Here's how the part is built. I have some questions about the finished solid (model axes, mm). Round coordinates to 2 decimals unless told otherwise and drop trailing zeros. Write each loop counter-clockwise with the first axis right and the second up, starting at its lowest first coordinate (ties: lowest second). Pieces come first, ordered by that corner, then holes. Notation, with made-up numbers: (-38.5, 57.25) - (1.5, 57.25) arc R32 ccw to (1.5, 83.25) - close; hole circle Ø11 at (-35, 54). An arc over 180 degrees is marked (long way). Return JSON: item names as keys, results as strings. Group by question number.
```python
from build123d import *

# Parameters (mm, degrees)
CROQUIS1_W              = 30
CROQUIS1_H              = 15
CROQUIS1_R              = 2.3
SALIENTE_EXTRUIR1_DEPTH = 16
CROQUIS2_W              = 120
CROQUIS2_H              = 50
CROQUIS2_R              = 3.5
SALIENTE_EXTRUIR2_DEPTH = 5
CROQUIS3_W              = 40
CROQUIS3_H              = 25
CROQUIS3_W_2            = 30
CROQUIS3_H_2            = 15
SALIENTE_EXTRUIR3_DEPTH = 4
CORTAR_EXTRUIR1_DEPTH   = 5
REDONDEO1_R             = 2


with BuildPart() as part:
    # Croquis1 → Saliente-Extruir1 (new body)
    with BuildSketch(Plane.XY):
        Rectangle(CROQUIS1_W, CROQUIS1_H)
        with Locations((6, 0)):
            Circle(CROQUIS1_R, mode=Mode.SUBTRACT)
        with Locations(Location((-6, 0, 0), (0, 0, 180))):
            Circle(CROQUIS1_R, mode=Mode.SUBTRACT)
    extrude(amount=SALIENTE_EXTRUIR1_DEPTH)

    # Croquis2 → Saliente-Extruir2 (add)
    with BuildSketch(Plane(origin=(0, 0, 0), x_dir=(-1, 0, 0), z_dir=(0, 0, -1))):
        with Locations((32.909933797, 0)):
            Rectangle(CROQUIS2_W, CROQUIS2_H)
        with Locations((-6, 0)):
            Circle(CROQUIS2_R, mode=Mode.SUBTRACT)
        with Locations((6, 0)):
            Circle(CROQUIS2_R, mode=Mode.SUBTRACT)
    extrude(amount=-SALIENTE_EXTRUIR2_DEPTH)

    # Croquis3 → Saliente-Extruir3 (add)
    with BuildSketch(Plane.XY.offset(5)):
        Rectangle(CROQUIS3_W, CROQUIS3_H)
        Rectangle(CROQUIS3_W_2, CROQUIS3_H_2, mode=Mode.SUBTRACT)
    extrude(amount=SALIENTE_EXTRUIR3_DEPTH)

    # Croquis4 → Cortar-Extruir1 (cut)
    with BuildSketch(Plane(origin=(0, 0, 0), x_dir=(-1, 0, 0), z_dir=(0, 0, -1))):
        with BuildLine():
            Line((6, 7.5), (-6, 7.5))
            ThreePointArc((-6, 7.5), (-13.5, 0), (-6, -7.5))
            Line((-6, -7.5), (6, -7.5))
            ThreePointArc((6, -7.5), (13.5, 0), (6, 7.5))
        make_face()
    extrude(amount=-CORTAR_EXTRUIR1_DEPTH, mode=Mode.SUBTRACT)

    # Redondeo1
    redondeo1_edges = [part.edges().sort_by_distance(p)[0] for p in [
        (27.090066203, -25, 2.5),
        (27.090066203, 25, 2.5),
        (-92.909933797, 25, 2.5),
        (-92.909933797, -25, 2.5),
        (20, -12.5, 7),
        (20, 12.5, 7),
        (-20, 12.5, 7),
        (-20, -12.5, 7),
        (15, -7.5, 12.5),
        (-15, -7.5, 12.5),
        (-15, 7.5, 12.5),
        (15, 7.5, 12.5),
    ]]
    fillet(redondeo1_edges, radius=REDONDEO1_R)


solid = part.part
```
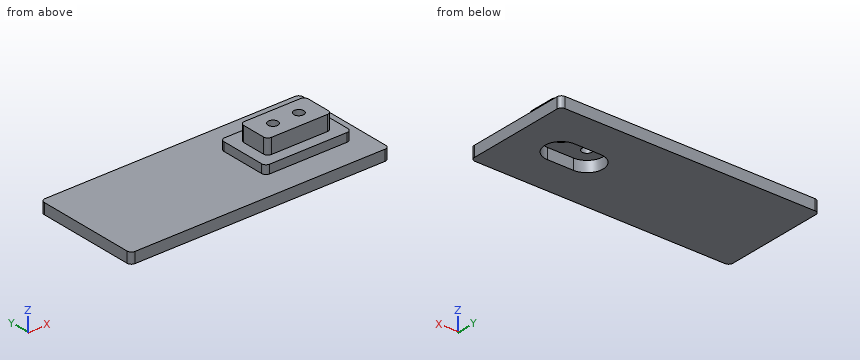
1) Will these pins go through, and if not, where does the flat tip stop? pin 1 Ø7.5 at (y, z) = (-2, 13.5) entering from +X; pin 2 Ø2 at (y, z) = (-1, 7.5) entering from +X; pin 3 Ø3.5 at (y, z) = (2.5, 13.5) entering from -X; pin 4 Ø4 at (x, y) = (6, 0) entering from +Z.
2) Imagine slicing it at C-C (x = -9.5). Please give me the cut outline in (y, z).
3) Imagine slicing it at A-A (y = 0). Please give me the cut outline in (x, z), plus the area to 3 significant figures.
4) I need wall thicknesses on line 1 along Y through (x, z) = (-6, 10.5); line 2 along Z through (x, y) = (-35, 23); line 3 along X through (y, z) = (-4, 14.75). Which ranges of each line are inside material? Lowest first, please.
5) Imagine slicing it at B-B (z = 10.75). Please give me the cut outline in (x, y), plus the area to 3 significant figures.
6) Imagine slicing it at D-D (x = -41.5). Please give me the cut outline in (y, z), plus the area to 3 significant figures.
Results found:
{
 "1": {"pin 1": "stops at x = 15", "pin 2": "stops at x = 20", "pin 3": "stops at x = -15", "pin 4": "passes through"},
 "2": {"outline": "(-25, 0) - (-6.63, 0) - (-6.63, 5) - (6.63, 5) - (6.63, 0) - (25, 0) - (25, 5) - (12.5, 5) - (12.5, 9) - (7.5, 9) - (7.5, 16) - (-7.5, 16) - (-7.5, 9) - (-12.5, 9) - (-12.5, 5) - (-25, 5) - close"},
 "3": {"outline": "(-92.91, 0) - (-13.5, 0) - (-13.5, 5) - (-8.3, 5) - (-8.3, 16) - (-15, 16) - (-15, 9) - (-20, 9) - (-20, 5) - (-92.91, 5) - close; (-3.7, 5) - (3.7, 5) - (3.7, 16) - (-3.7, 16) - close; (8.3, 5) - (13.5, 5) - (13.5, 0) - (27.09, 0) - (27.09, 5) - (20, 5) - (20, 9) - (15, 9) - (15, 16) - (8.3, 16) - close", "area": "734 mm²"},
 "4": {"line 1": "y = -7.5 to -2.3, 2.3 to 7.5", "line 2": "z = 0 to 5", "line 3": "x = -15 to 15"},
 "5": {"outline": "(-15, -5.5) arc R2 ccw to (-13, -7.5) - (13, -7.5) arc R2 ccw to (15, -5.5) - (15, 5.5) arc R2 ccw to (13, 7.5) - (-13, 7.5) arc R2 ccw to (-15, 5.5) - close; hole circle Ø4.6 at (-6, 0); hole circle Ø4.6 at (6, 0)", "area": "413 mm²"},
 "6": {"outline": "(-25, 0) - (25, 0) - (25, 5) - (-25, 5) - close", "area": "250 mm²"}
}
